Read the model definition and answer for the solid it produces. Units are mm, in the model's axes. A direction names the side the tool comes from. Give positions to 0.01 mm unless a question says otherwise; leave off trailing zeros. Order: outer loops, then holes, each group sorted by start corner. A loop starts at its lowest first (then second) coordinate and runs counter-clockwise, first axis right, second up.
Item 1: A cutting plane is placed at C-C (z = -17). Write down the section's boundary in (x, y).
Item 2: Which of the six approach directions +Z, -Z, +X, -X, +Y, -Y give full straight-line access (tool end or side, diameter ignored) to faces 1 (the face through (-1, 0, -96)), 2 (the face through (-80.086, 0.165, 1.521)), 3 (the face through (77.908, 0.601, 1.521))?
Item 3: Find the intervals of material crossed by line 1 along Z through (x, y) = (55, -19); line 2 along Z through (x, y) = (32, 2.5); line 3 along X through (y, z) = (-18, -76), in increasing order.
Item 4: Given pin 1 Ø4 at (x, z) = (87.5, -48) entering from -Y; pin 2 Ø4 at (x, z) = (66.5, -7.5) entering from +Y, each flat-ended and moving along its own axis, determine where each tip first touches the part or whether it passes through.
Item 5: A cutting plane is placed at B-B (x = 50). Write down the section's boundary in (y, z).
Item 6: The mould has two halves that part along Y. Classify faces 4 (the face through (-1, 0, 0)), 5 (the face through (72.423, 1.126, -97.521)), 6 (the face through (-1, -20.5, -13)): +Y half, -Y half, draft (parallel to the pull), parting line (faces both ways), or undercut.
Item 7: A cutting plane is placed at A-A (y = -15.5). Write down the section's boundary in (x, z).
from build123d import *

# Parameters (mm, degrees)
SKETCH_1_W          = 180
SKETCH_1_H          = 35
EXTRUDE_1_DEPTH     = 3
SKETCH_2_R          = 3.75
SKETCH_2_R_2        = 2
CUT_EXTRUDE_1_DEPTH = 3
SKETCH_3_R          = 1.1
CUT_EXTRUDE_2_DEPTH = 3
SKETCH_4_W          = 180
SKETCH_4_H          = 102
EXTRUDE_2_DEPTH     = 3
SKETCH_5_W          = 180
SKETCH_5_H          = 3
EXTRUDE_3_DEPTH     = 35
SKETCH_6_R          = 3.75
SKETCH_6_R_2        = 2
SKETCH_6_R_3        = 1.1
SKETCH_6_R_4        = 0.981653735
CUT_EXTRUDE_3_DEPTH = 35
SKETCH_9_W          = 115.5
SKETCH_9_H          = 66.5
CUT_EXTRUDE_4_DEPTH = 10
SKETCH_10_R         = 1.25
CUT_EXTRUDE_5_DEPTH = 10
SKETCH_11_R         = 1.25
SKETCH_11_W         = 17
SKETCH_11_H         = 9
CUT_EXTRUDE_6_DEPTH = 10
SKETCH_12_R         = 1.25
CUT_EXTRUDE_7_DEPTH = 10


with BuildPart() as part:
    # 스케치1 → 보스-돌출1 (new body)
    with BuildSketch(Plane.XY):
        Rectangle(SKETCH_1_W, SKETCH_1_H)
    extrude(amount=EXTRUDE_1_DEPTH)

    # 스케치2 → 컷-돌출1 (cut)
    with BuildSketch(Plane.XY.offset(3)):
        with Locations((-76.33997629, 0)):
            Circle(SKETCH_2_R)
        with Locations((76, 0)):
            Circle(SKETCH_2_R_2)
    extrude(amount=-CUT_EXTRUDE_1_DEPTH, mode=Mode.SUBTRACT)

    # 스케치3 → 컷-돌출2 (cut)
    with BuildSketch(Plane.XY.offset(3)):
        with Locations((-76.33997629, 8.5)):
            Circle(SKETCH_3_R)
        with Locations((-76.33997629, -8.5)):
            Circle(SKETCH_3_R)
        with Locations((-84.83997629, 0)):
            Circle(SKETCH_3_R)
        with Locations((-67.83997629, 0)):
            Circle(SKETCH_3_R)
        with Locations((76, 8.5)):
            Circle(SKETCH_3_R)
        with Locations((76, -8.5)):
            Circle(SKETCH_3_R)
        with Locations((67.5, 0)):
            Circle(SKETCH_3_R)
        with Locations((84.5, 0)):
            Circle(SKETCH_3_R)
    extrude(amount=-CUT_EXTRUDE_2_DEPTH, mode=Mode.SUBTRACT)

    # 스케치4 → 보스-돌출2 (add)
    with BuildSketch(Plane.XZ.offset(17.5)):
        with Locations((0, -48)):
            Rectangle(SKETCH_4_W, SKETCH_4_H)
    extrude(amount=EXTRUDE_2_DEPTH)

    # 스케치5 → 보스-돌출3 (add)
    with BuildSketch(Plane(origin=(0, -17.5, 0), x_dir=(1, 0, 0), z_dir=(0, 1, 0))):
        with Locations((0, 97.5)):
            Rectangle(SKETCH_5_W, SKETCH_5_H)
    extrude(amount=EXTRUDE_3_DEPTH)

    # 스케치6 → 컷-돌출3 (cut)
    with BuildSketch(Plane(origin=(0, 0, -99), x_dir=(-1, 0, 0), z_dir=(0, 0, -1))):
        with Locations((-76, 0)):
            Circle(SKETCH_6_R)
        with Locations((76.33997629, 0)):
            Circle(SKETCH_6_R_2)
        with Locations((-76, -8.5)):
            Circle(SKETCH_6_R_3)
        with Locations((-67.5, 0)):
            Circle(SKETCH_6_R_3)
        with Locations((-76, 8.5)):
            Circle(SKETCH_6_R_4)
        with Locations((-84.5, 0)):
            Circle(SKETCH_6_R_3)
        with Locations((84.83997629, 0)):
            Circle(SKETCH_6_R_3)
        with Locations((76.33997629, 8.5)):
            Circle(SKETCH_6_R_3)
        with Locations((67.83997629, 0)):
            Circle(SKETCH_6_R_3)
        with Locations((76.33997629, -8.5)):
            Circle(SKETCH_6_R_3)
    extrude(amount=-CUT_EXTRUDE_3_DEPTH, mode=Mode.SUBTRACT)

    # 스케치9 → 컷-돌출4 (cut)
    with BuildSketch(Plane(origin=(0, -17.5, 0), x_dir=(1, 0, 0), z_dir=(0, 1, 0))):
        with Locations((0, 48)):
            Rectangle(SKETCH_9_W, SKETCH_9_H)
    extrude(amount=-CUT_EXTRUDE_4_DEPTH, mode=Mode.SUBTRACT)

    # 스케치10 → 컷-돌출5 (cut)
    with BuildSketch(Plane.XZ.offset(20.5)):
        with Locations((-55, -8)):
            Circle(SKETCH_10_R)
        with Locations((55, -8)):
            Circle(SKETCH_10_R)
        with Locations((55, -88)):
            Circle(SKETCH_10_R)
        with Locations((-55, -88)):
            Circle(SKETCH_10_R)
    extrude(amount=-CUT_EXTRUDE_5_DEPTH, mode=Mode.SUBTRACT)

    # 스케치11 → 컷-돌출6 (cut)
    with BuildSketch(Plane.XZ.offset(20.5)):
        with Locations((21, -8)):
            Circle(SKETCH_11_R)
        with Locations((-21, -8)):
            Circle(SKETCH_11_R)
        with Locations((21, -88)):
            Circle(SKETCH_11_R)
        with Locations((-21, -88)):
            Circle(SKETCH_11_R)
        with Locations((38, -88)):
            Rectangle(SKETCH_11_W, SKETCH_11_H)
        with Locations((-38, -88)):
            Rectangle(SKETCH_11_W, SKETCH_11_H)
        with Locations((38, -8)):
            Rectangle(SKETCH_11_W, SKETCH_11_H)
        with Locations((-38, -8)):
            Rectangle(SKETCH_11_W, SKETCH_11_H)
    extrude(amount=-CUT_EXTRUDE_6_DEPTH, mode=Mode.SUBTRACT)

    # 스케치12 → 컷-돌출7 (cut)
    with BuildSketch(Plane(origin=(0, -17.5, 0), x_dir=(1, 0, 0), z_dir=(0, 1, 0))):
        with Locations((-87.5, 86)):
            Circle(SKETCH_12_R)
        with Locations((-87.5, 67)):
            Circle(SKETCH_12_R)
        with Locations((-87.5, 48)):
            Circle(SKETCH_12_R)
        with Locations((-87.5, 29)):
            Circle(SKETCH_12_R)
        with Locations((-87.5, 10)):
            Circle(SKETCH_12_R)
        with Locations((87.328433312, 86)):
            Circle(SKETCH_12_R)
        with Locations((87.5, 67)):
            Circle(SKETCH_12_R)
        with Locations((87.5, 48)):
            Circle(SKETCH_12_R)
        with Locations((87.5, 29)):
            Circle(SKETCH_12_R)
        with Locations((87.5, 10)):
            Circle(SKETCH_12_R)
    extrude(amount=-CUT_EXTRUDE_7_DEPTH, mode=Mode.SUBTRACT)


solid = part.part
Response values:
1. outline: (-90, -20.5) - (-57.75, -20.5) - (-57.75, -17.5) - (-90, -17.5) - close; (57.75, -20.5) - (90, -20.5) - (90, -17.5) - (57.75, -17.5) - close
2. face 1: +X, -X, +Y
2. face 2: +Z
2. face 3: +Z, -Z
3. line 1: z = -99 to -89.25, -86.75 to -81.25, -14.75 to -9.25, -6.75 to 3
3. line 2: z = -99 to -96, 0 to 3
3. line 3: x = -90 to -57.75, 57.75 to 90
4. pin 1: stops at y = -20.5
4. pin 2: stops at y = -17.5
5. outline: (-20.5, -99) - (17.5, -99) - (17.5, -96) - (-17.5, -96) - (-17.5, -81.25) - (-20.5, -81.25) - close; (-20.5, -14.75) - (-17.5, -14.75) - (-17.5, 0) - (17.5, 0) - (17.5, 3) - (-20.5, 3) - close
6. face 4: draft
6. face 5: undercut
6. face 6: -Y half
7. outline: (-90, -99) - (90, -99) - (90, -96) - (-90, -96) - close; (-90, 0) - (90, 0) - (90, 3) - (-90, 3) - close
